```python
from build123d import *

# Parameters (mm, degrees)
BOSS_EXTRUDE1_DEPTH = 15


with BuildPart() as part:
    # Sketch1 → Boss-Extrude1 (new body)
    with BuildSketch(Plane.XY):
        with BuildLine():
            Line((0, 0), (13.001019729, 0))
            Line((13.001019729, 0), (12.974193154, 52.70215653))
            Line((12.974193154, 52.70215653), (10.974193413, 52.701138486))
            Line((10.974193413, 52.701138486), (10.997204677, 7.494352092))
            ThreePointArc((10.997204677, 7.494352092), (9.725689165, 3.977520123), (6.497205517, 2.090259641))
            ThreePointArc((6.497205517, 2.090259641), (3.270511139, 3.975372484), (1.997206357, 7.488761443))
            Line((1.997206357, 7.488761443), (1.99083734, 20.001015713))
            Line((1.99083734, 20.001015713), (-0.009162401, 19.999997668))
            Line((-0.009162401, 19.999997668), (0, 2))
            Line((0, 2), (0, 0))
        make_face()
    extrude(amount=BOSS_EXTRUDE1_DEPTH)


solid = part.part
```
Geometry check sheet. Reference: the model listing, model coordinates, mm. A direction names the side the tool comes from. Round coordinates to 2 decimals unless told otherwise and drop trailing zeros. Loops run counter-clockwise (first coordinate to the right, second up) from the corner with the lowest first, then second, coordinate; pieces in that order, holes last. Notation, with made-up numbers: (30, 35) -> (50, 35) arc R20 ccw to (50, 42) -> close; hole circle Ø4 at (11, 23). An arc over 180 degrees is marked (long way). Use a Markdown table: item, result.
(1) Sectioned sample at D-D (x = 9.25). Enter the section's corners in (y, z).
Calculated:
| item | result |
|---|---|
| outline | (0, 0) -> (3.47, 0) -> (3.47, 15) -> (0, 15) -> close |
(2) Sectioned sample at C-C (y = 4). Enter the section's corners in (x, z).
Calculated:
| item | result |
|---|---|
| outline | (0, 0) -> (3.25, 0) -> (3.25, 15) -> (0, 15) -> close; (9.74, 0) -> (13, 0) -> (13, 15) -> (9.74, 15) -> close |
(3) Scan lines: probe 1 along X at (y, z) = (10, 10.75); probe 2 along Y at (x, z) = (1.5, 4); probe 3 along X at (y, z) = (49, 4.25). Record each from-to range of solid material in increasing order.
Calculated:
| item | result |
|---|---|
| probe 1 | 0 to 2, 11 to 13 |
| probe 2 | 0 to 20 |
| probe 3 | 10.98 to 12.98 |
(4) Set-up check for faces 1 (the flat face through (6, 0, 7)), 2 (the cylindrical face through (3.305, 3.935, 7.395)): record each of +Z, -Z, +X, -X, +Y, -Y from which the full face is reachable in a straight line by a thin tool's end or side.
Calculated:
| item | result |
|---|---|
| face 1 | +Z, -Z, +X, -X, -Y |
| face 2 | +Z, -Z, +Y |
(5) Go/stop test with flat-tipped pins: P1, Ø0.6, axis at y = 1, z = 6.5, coming from the -X side; P2, Ø1.5, axis at x = 7.5, z = 8, coming from the +Y side; P3, Ø1, axis at x = 2, z = 2.5, coming from the +Y side. Record where each tip stops, or that it passes through.
Calculated:
| item | result |
|---|---|
| P1 | x = 0 |
| P2 | y = 2.73 |
| P3 | y = 20 |
(6) Sectioned sample at A-A (z = 12.75). Enter the section's corners in (x, y).
Calculated:
| item | result |
|---|---|
| outline | (-0.01, 20) -> (0, 2) -> (0, 0) -> (13, 0) -> (12.97, 52.7) -> (10.97, 52.7) -> (11, 7.49) arc R5.49 cw to (6.5, 2.09) arc R5.49 cw to (2, 7.49) -> (1.99, 20) -> close |
(7) Sectioned sample at B-B (y = 16). Enter the section's corners in (x, z).
Calculated:
| item | result |
|---|---|
| outline | (-0.01, 0) -> (1.99, 0) -> (1.99, 15) -> (-0.01, 15) -> close; (10.99, 0) -> (12.99, 0) -> (12.99, 15) -> (10.99, 15) -> close |
